Read the model definition and answer for the solid it produces. Units are mm, in the model's axes. A direction names the side the tool comes from. Give positions to 0.01 mm unless a question says otherwise; leave off trailing zeros. Order: outer loops, then holes, each group sorted by start corner. A loop starts at its lowest first (then second) coordinate and runs counter-clockwise, first axis right, second up.
```python
from build123d import *

# Parameters (mm, degrees)
SKETCH_W               = 16
SKETCH_H               = 31
PAD_DEPTH              = 15
SKETCH001_R            = 2.5
POCKET_DEPTH           = 5
SKETCH002_R            = 3
PAD001_DEPTH           = 1.65
LINEARPATTERN_COUNT    = 2
LINEARPATTERN_PITCH    = 6.3
LINEARPATTERN001_COUNT = 2
LINEARPATTERN001_PITCH = 6.3
FILLET_R               = 1
FILLET001_R            = 1
FILLET002_R            = 1
FILLET003_R            = 1
FILLET004_R            = 1
FILLET005_R            = 1


with BuildPart() as part:
    # Sketch → Pad (new body)
    with BuildSketch(Plane.XZ):
        Polygon((0, 0), (-44, 0), (-44, -41), (-24, -41), (-24, -5), (0, -5), align=None)
        with Locations((-34, -20.5)):
            Rectangle(SKETCH_W, SKETCH_H, mode=Mode.SUBTRACT)
    pad = extrude(amount=PAD_DEPTH)

    # Mirrored: Pad across Sketch V_Axis
    add(pad.mirror(Plane(origin=(0, 0, 0), x_dir=(0, -1, 0), z_dir=(1, 0, 0))))

    # Sketch001 (on Face11 of Mirrored) → Pocket (cut)
    with BuildSketch(Plane(origin=(0, 0, -36), x_dir=(-1, 0, 0), z_dir=(0, 0, 1))):
        with Locations((-34, 7.5)):
            Circle(SKETCH001_R)
    pocket = extrude(amount=-POCKET_DEPTH, mode=Mode.SUBTRACT)

    # Mirrored001: Pocket across Sketch001 V_Axis
    add(pocket.mirror(Plane(origin=(0, 0, -36), x_dir=(0, 0, 1), z_dir=(-1, 0, 0))), mode=Mode.SUBTRACT)

    # Sketch002 → Pad001 (join, symmetric)
    with BuildSketch(Plane.YZ):
        with BuildLine():
            Line((-15, 0), (0, 0))
            Line((0, 0), (0, 12))
            ThreePointArc((0, 12), (-7.5, 19.163278), (-15, 12))
            Line((-15, 12), (-15, 0))
        make_face()
        with Locations((-7.5, 11.655364)):
            Circle(SKETCH002_R, mode=Mode.SUBTRACT)
    pad001 = extrude(amount=PAD001_DEPTH, both=True)

    # LinearPattern: Pad001 ×2
    with Locations(*[(i * LINEARPATTERN_PITCH, 0, 0) for i in range(1, LINEARPATTERN_COUNT)]):
        add(pad001)

    # LinearPattern001: Pad001 ×2
    with Locations(*[(-i * LINEARPATTERN001_PITCH, 0, 0) for i in range(1, LINEARPATTERN001_COUNT)]):
        add(pad001)

    # Fillet
    fillet_edges = [part.edges().sort_by_distance(p)[0] for p in [
        (25.975, 0, 0),
    ]]
    fillet(fillet_edges, radius=FILLET_R)

    # Fillet001
    fillet001_edges = [part.edges().sort_by_distance(p)[0] for p in [
        (-25.975, 0, 0),
    ]]
    fillet(fillet001_edges, radius=FILLET001_R)

    # Fillet002
    fillet002_edges = [part.edges().sort_by_distance(p)[0] for p in [
        (25.975, -15, 0),
    ]]
    fillet(fillet002_edges, radius=FILLET002_R)

    # Fillet003
    fillet003_edges = [part.edges().sort_by_distance(p)[0] for p in [
        (-25.975, -15, 0),
    ]]
    fillet(fillet003_edges, radius=FILLET003_R)

    # Fillet004
    fillet004_edges = [part.edges().sort_by_distance(p)[0] for p in [
        (-44, -7.5, 0),
    ]]
    fillet(fillet004_edges, radius=FILLET004_R)

    # Fillet005
    fillet005_edges = [part.edges().sort_by_distance(p)[0] for p in [
        (44, -7.5, 0),
    ]]
    fillet(fillet005_edges, radius=FILLET005_R)


solid = part.part
```
1) The part is cut by section C-C on x = -34. Determine the outline of the cut face in (y, z).
Final values:
outline: (-15, -41) - (-10, -41) - (-10, -36) - (-15, -36) - close; (-15, -5) - (0, -5) - (0, -1) arc R1 ccw to (-1, 0) - (-14, 0) arc R1 ccw to (-15, -1) - close; (-5, -41) - (0, -41) - (0, -36) - (-5, -36) - close
2) For a pull along X with two mould halves and no side action, classify faces 4 (the face through (-7.95, -8, 7)), 5 (the face through (-24, -7, -23)), 6 (the face through (0.2, -15, -4.6)), 7 (the face through (7.95, -8, 7)) as released by +X, released by -X, zero draft, split by the parting line, or undercut.
Final values:
face 4: released by -X
face 5: undercut
face 6: zero draft
face 7: released by +X
3) The part is cut by section A-A on z = -37. Determine the outline of the cut face in (x, y).
Final values:
outline: (-44, -14) arc R1 ccw to (-43, -15) - (-24, -15) - (-24, 0) - (-43, 0) arc R1 ccw to (-44, -1) - close; (24, -15) - (43, -15) arc R1 ccw to (44, -14) - (44, -1) arc R1 ccw to (43, 0) - (24, 0) - close; hole circle Ø5 at (-34, -7.5); hole circle Ø5 at (34, -7.5)
4) A tool of negligible diameter and unlimited length cuts with its end or side. For faces 1 (the face through (1.65, -8, 8)), 2 (the face through (-26, -7, 0)), 3 (the face through (26, -7, -21)), from which of +Z, -Z, +X, -X, +Y, -Y can it reach the whole face along a straight path? Write none if from no direction.
Final values:
face 1: +Z, +Y, -Y
face 2: +Z, -X, +Y, -Y
face 3: +Y, -Y
5) Consider L1, parallel to X at y = -6.5, z = -22.5; L2, parallel to X at y = -7.5, z = -39.45; L3, parallel to X at y = -2, z = 16. Determine where each line is inside the solid, lowest interval first.
Final values:
L1: x = -44 to -42, -26 to -24, 24 to 26, 42 to 44
L2: x = -44 to -36.5, -31.5 to -24, 24 to 31.5, 36.5 to 44
L3: x = -7.95 to -4.65, -1.65 to 1.65, 4.65 to 7.95
6) Given pin 1 (4.5 mm diameter, centred on y = -8.5, z = 7.5, fed in from -X); pin 2 (2 mm diameter, centred on x = -18, y = -8.5, fed in from +Z); pin 3 (4.5 mm diameter, centred on y = -7, z = 12.5, fed in from +X), each flat-ended and moving along its own axis, determine where each tip first touches the part or whether it passes through.
Final values:
pin 1: stops at x = -7.95
pin 2: stops at z = 0
pin 3: stops at x = 7.95
7) The part is cut by section B-B on z = -22. Determine the outline of the cut face in (x, y).
Final values:
outline: (-44, -14) arc R1 ccw to (-43, -15) - (-42, -15) - (-42, 0) - (-43, 0) arc R1 ccw to (-44, -1) - close; (-26, -15) - (-24, -15) - (-24, 0) - (-26, 0) - close; (24, -15) - (26, -15) - (26, 0) - (24, 0) - close; (42, -15) - (43, -15) arc R1 ccw to (44, -14) - (44, -1) arc R1 ccw to (43, 0) - (42, 0) - close
8) The part is cut by section D-D on y = -7.5. Count the separate pieces of the cut face and the enclosed holes in it, and give its area (3 significant figures).
Final values:
separate pieces: 4
enclosed holes: 0
area: 968 mm2
